Autodesk Inventor part; units mm, degrees
ref_plane "YZ Plane" through (0, 0, 0) normal (1, 0, 0) x (0, 1, 0)
ref_plane "XZ Plane" through (0, 0, 0) normal (0, 1, 0) x (-1, 0, 0)
ref_plane "XY Plane" through (0, 0, 0) normal (0, 0, 1) x (1, 0, 0)
sketch "スケッチ2" plane through (0, 0, 0) normal (1, 0, 0) x (0, 1, 0)
  line L0 (25, 10) -> (-25, 10)
  line L1 (-25, 10) -> (-25, -10)
  line L2 (-25, -10) -> (25, -10)
  line L3 (25, -10) -> (25, 10)
  line L4 (25, 10) -> (-25, -10) construction
  line L5 (-25, 10) -> (25, -10) construction
  point P0 (0, 0)
  dimension "d4" = 50
  dimension "d5" = 20
extrude "押し出し2" add sketch "スケッチ2" along normal mid plane 500
sketch "スケッチ3" plane through (-250, -25, 10) normal (0, 0, 1) x (1, 0, 0)
  circle A0 centre (250, 25) radius 5
  dimension "d8" = 10
extrude "押し出し3" add sketch "スケッチ3" along normal blind 2
fillet "フィレット1" radius 2 2 edges at (250, 0, -10) (-250, 0, -10)
sketch "スケッチ4" plane through (250, 0, 0) normal (1, 0, 0) x (0, 0, -1)
  line L0 (-6, 21) -> (6, 21)
  line L1 (6, 21) -> (6, -21)
  line L2 (6, -21) -> (-6, -21)
  line L3 (-6, -21) -> (-6, 21)
  line L4 (-6, 21) -> (6, -21) construction
  line L5 (6, 21) -> (-6, -21) construction
  point P0 (0, 0)
  dimension "d12" = 12
  dimension "d13" = 42
extrude "押し出し4" cut sketch "スケッチ4" against normal through all
sketch "スケッチ6" plane through (-250, -25, 10) normal (0, -1, 0) x (1, 0, 0)
  line L0 (4, -2) -> (496, -2)
  line L1 (496, -2) -> (496, -18)
  line L2 (496, -18) -> (4, -18)
  line L3 (4, -18) -> (4, -2)
  line L4 (4, -2) -> (496, -18) construction
  line L5 (496, -2) -> (4, -18) construction
  point P0 (250, -10)
  dimension "d16" = 492
  dimension "d17" = 16
extrude "押し出し5" cut sketch "スケッチ6" against normal through all
properties part number "hashi1shado"
Here's how the part is built. I have some questions about the finished solid (model axes, mm). A direction names the side the tool comes from. Coordinates: 2 decimals unless noted, no trailing zeros. Order: outer loops, then holes, each group sorted by start corner. A loop starts at its lowest first (then second) coordinate and runs counter-clockwise, first axis right, second up. Notation, with made-up numbers: (66, -31.5) - (88, -31.5) arc R17 cw to (88, -0.5) - close; hole circle Ø4 at (-12.5, 29.25). An arc over 180 degrees is marked (long way). Use CSV: the item, a comma, the result in double quotes. Start each with the question number.
1. Suppose I cut it at C-C on y = 0. List the corners of the cut face in (x, z) for me, then the cut area to 3 significant figures.
2. I'm going to push flat-ended pins straight in: pin 1 (1.5 mm diameter, centred on x = -25, y = 0.5, fed in from +Z); pin 2 (10 mm diameter, centred on y = 2, z = 0, fed in from +X). Where does each tip first touch, or does it pass through?
3. Please list where these lines run through material, in increasing order: line 1 (Z direction, x = -46, y = 3.5); line 2 (X direction, y = 1, z = 6.75). Write a range as from..to.
4. Suppose I cut it at B-B on x = 40.5. List the corners of the cut face in (y, z) for me, then the cut area to 3 significant figures.
5. If we mould it in two halves opening along Z, with no side actions, what happens to faces 1 (the face through (-246, 0, 7)), 2 (the face through (246, 0, -7)), 3 (the face through (-4, 6, 10)), 4 (the face through (17.4, 25, -8.2))? For each: +Z half, -Z half, draft (parallel to the pull), parting line (faces both ways), or undercut.
6. Suppose I cut it at A-A on z = -0.75. List the corners of the cut face in (x, y) for me.
7. For faces 5 (the face through (17.4, -25, 8.2)), 6 (the face through (-3, 0, 8)), 7 (the face through (-1.08, 4.88, 10.99)), which set-ups out of +Z, -Z, +X, -X, +Y, -Y let a thin tool reach every point of the face, with its end or its side?
Output:
1,outline,"(-250, -8) arc R2 ccw to (-248, -10) - (248, -10) arc R2 ccw to (250, -8) - (250, -6) - (246, -6) - (246, -8) - (-246, -8) - (-246, -6) - (-250, -6) - close; (-250, 6) - (-246, 6) - (-246, 8) - (246, 8) - (246, 6) - (250, 6) - (250, 10) - (5, 10) - (5, 12) - (-5, 12) - (-5, 10) - (-250, 10) - close"
1,area,"2,050 mm2"
2,pin 1,"stops at z = 10"
2,pin 2,"passes through"
3,line 1,"z = -10..-8, 8..10"
3,line 2,"x = -250..-246, 246..250"
4,outline,"(-25, -10) - (25, -10) - (25, -8) - (-25, -8) - close; (-25, 8) - (25, 8) - (25, 10) - (-25, 10) - close"
4,area,"200 mm2"
5,face 1,"undercut"
5,face 2,"undercut"
5,face 3,"+Z half"
5,face 4,"draft"
6,outline,"(-250, -25) - (-246, -25) - (-246, -21) - (-250, -21) - close; (-250, 21) - (-246, 21) - (-246, 25) - (-250, 25) - close; (246, -25) - (250, -25) - (250, -21) - (246, -21) - close; (246, 21) - (250, 21) - (250, 25) - (246, 25) - close"
7,face 5,"+Z, -Z, +X, -X, -Y"
7,face 6,"+Y, -Y"
7,face 7,"+Z"
